from build123d import *

# Parameters (mm, degrees)
EYE_SKETCH_W = 7.6
EYE_SKETCH_H = 4


with BuildPart() as part:
    # Eye Sketch → Eye (revolve)
    with BuildSketch(Plane.XY, mode=Mode.PRIVATE) as eye_sk:
        with Locations((0, 4)):
            Rectangle(EYE_SKETCH_W, EYE_SKETCH_H)
    revolve(eye_sk.sketch.rotate(Axis((-3000, 0, 0), (1, 0, 0)), 90), axis=Axis((-3000, 0, 0), (1, 0, 0)))

    # Shank Sketch → Shank (revolve)
    with BuildSketch(Plane.XY, mode=Mode.PRIVATE) as shank_sk:
        Polygon((0, 5), (2.5, 5), (2.5, 20), (1.25, 20), (1.25, 10), (0, 10), align=None)
    revolve(shank_sk.sketch.rotate(Axis((0, -5, 0), (0, 1, 0)), 90), axis=Axis((0, -5, 0), (0, 1, 0)))


solid = part.part
The model under review builds one solid part; all positions refer to its coordinate system, in mm. A direction names the side the tool comes from. Give positions to 0.01 mm unless a question says otherwise; leave off trailing zeros. Loops run counter-clockwise (first coordinate to the right, second up) from the corner with the lowest first, then second, coordinate; pieces in that order, holes last. Notation, with made-up numbers: (39.5, 75.5) -> (60.5, 75.5) arc R20 cw to (60.5, 82.5) -> close; hole circle Ø3 at (-35.75, -25.5). An arc over 180 degrees is marked (long way). Put each result on its own line as item: value. Start each with the question number.
1. We need section B-B on y = 0. State the section outline as (x, z) points.
2. Wall thickness on probe 1 along X at (y, z) = (14.25, 0); probe 2 along Z at (x, y) = (-1, -1.25); probe 3 along Z at (x, y) = (-0.5, 13): over which ranges is each line inside the solid? List them lowest first.
3. Clearance check with flat-ended pins moving along their axes: P1, Ø1, axis at x = -0.5, y = 3.5, coming from the +Z side; P2, Ø1.5, axis at x = -1.5, y = 2, coming from the -Z side; P3, Ø3, axis at x = -1, z = 4, coming from the -Y side. State where each tip first meets the part, or that it passes through.
4. We need section A-A on z = 0. State the section outline as (x, y) points.
5. We need section D-D on y = 14.75. State the section outline as (x, z) points.
6. Mouldability with a two-part tool opening along X and no side actions: class faces 1 (the face through (-3.8, 0, -3)), 2 (the face through (3.8, 0, -3)), 3 (the face through (-0.05, 14.93, 1.25)) as released by +X, released by -X, zero draft, split by the parting line, or undercut.
7. We need section C-C on x = 0. State the section outline as (y, z) points, then the cut area to 3 significant figures.
8. For faces 4 (the face through (-0.1, 12.8, 2.5)), 5 (the face through (-1, 20, -1)), list the 3-axis set-ups (+Z, -Z, +X, -X, +Y, -Y) from which the entire face can be reached by the end or side of a thin tool; tool diameter is ignored.
Determined:
1. outline: (-3.8, -6) -> (3.8, -6) -> (3.8, -2) -> (-3.8, -2) -> close; (-3.8, 2) -> (3.8, 2) -> (3.8, 6) -> (-3.8, 6) -> close
2. probe 1: -2.5 to -1.25, 1.25 to 2.5
2. probe 2: -5.87 to -1.56, 1.56 to 5.87
2. probe 3: -2.45 to -1.15, 1.15 to 2.45
3. P1: z = 5.2
3. P2: z = -5.87
3. P3: y = -5.45
4. outline: (-3.8, -6) -> (3.8, -6) -> (3.8, -2) -> (-3.8, -2) -> close; (-3.8, 2) -> (3.8, 2) -> (3.8, 6) -> (2.5, 6) -> (2.5, 20) -> (1.25, 20) -> (1.25, 10) -> (-1.25, 10) -> (-1.25, 20) -> (-2.5, 20) -> (-2.5, 6) -> (-3.8, 6) -> close
5. outline: circle Ø5 at (0, 0); hole circle Ø2.5 at (0, 0)
6. face 1: released by -X
6. face 2: released by +X
6. face 3: undercut
7. outline: (5.45, -2.5) -> (20, -2.5) -> (20, -1.25) -> (10, -1.25) -> (10, 1.25) -> (20, 1.25) -> (20, 2.5) -> (5.45, 2.5) arc R6 ccw (long way) to start; hole circle Ø4 at (0, 0)
7. area: 146 mm^2
8. face 4: +Y
8. face 5: +Z, -Z, +X, -X, +Y
